Can you work these out from the model? Positions are in its coordinate system, mm. Face numbers are marked on the shaded views. Coordinates: 2 decimals unless noted, no trailing zeros. Write each loop counter-clockwise with the first axis right and the second up, starting at its lowest first coordinate (ties: lowest second). Pieces come first, ordered by that corner, then holes. Notation, with made-up numbers: (-2, 2) - (28, 2) arc R33 ccw to (28, 40) - close; hole circle Ø7 at (59, 23.5). An arc over 180 degrees is marked (long way). Use one line per item in the form item = value. Start each with the question number.
(1) If I drill on probe 1 along Y at (x, z) = (-29, 8); probe 2 along X at (y, z) = (11.5, 7.5); probe 3 along Z at (x, y) = (13, -8.5), over which ranges is the centre line in solid material (lowest first)? Write a range as from..to.
(2) If we section it at C-C on z = 12: Please give me the cut outline in (x, y), then the cut area to 3 significant figures.
(3) If we section it at A-A on z = 7.25: Give the number of separate pieces and of enclosed holes in the cut face, then the cut area to 3 significant figures.
(4) For pin 1 Ø3 at (y, z) = (17, 3.5) entering from -X; pin 2 Ø2 at (x, y) = (27.5, -15.5) entering from +Z; pin 3 Ø2 at (x, y) = (28.5, 11) entering from +Z; pin 4 Ø6 at (y, z) = (14.5, 13.5) entering from -X, each with a flat end and sliding along its axis, tell me the tip position at first contact or that it passes through.
(5) Thinking about a two-plate mould opening in X: for the marked faces 1, 2 and 3, which applies, pulls with the +X half, pulls with the -X half, needs draft (parallel to the pull), parting line crosses it, or undercut?
```python
from build123d import *

# Parameters (mm, degrees)
F2_DEPTH = 3
F1_R     = 2.5
F1_R_2   = 1.25
F3_DEPTH = 10
F4_SIZE2 = 3
F4_SIZE  = 2
F5_R     = 2.99999
F7_W     = 10
F7_H     = 18
F8_DEPTH = 4
F10_SIZE = 1


# Not quite as in the source:
# - a fillet or chamfer is up to 0.001 mm smaller than in the source, because OpenCascade refuses the exact size


with BuildPart() as f2:
    # F0 (on Top) → F2 (new body)
    with BuildSketch(Plane.XY):
        with BuildLine():
            ThreePointArc((46, 18), (43.0710678119, 25.0710678119), (36, 28))
            Line((36, 28), (-36, 28))
            ThreePointArc((-36, 28), (-43.0710678119, 25.0710678119), (-46, 18))
            Line((-46, 18), (-46, -18))
            ThreePointArc((-46, -18), (-43.0710678119, -25.0710678119), (-36, -28))
            Line((-36, -28), (36, -28))
            ThreePointArc((36, -28), (43.0710678119, -25.0710678119), (46, -18))
            Line((46, -18), (46, 18))
        make_face()
    extrude(amount=F2_DEPTH)

    # F1 (on Top) → F3 (join)
    with BuildSketch(Plane.XY):
        with Locations((-29, 11.5)):
            Circle(F1_R)
        with Locations((-29, 11.5)):
            Circle(F1_R_2, mode=Mode.SUBTRACT)
        with Locations((29, 11.5)):
            Circle(F1_R)
        with Locations((29, 11.5)):
            Circle(F1_R_2, mode=Mode.SUBTRACT)
        with Locations((-29, -11.5)):
            Circle(F1_R)
        with Locations((-29, -11.5)):
            Circle(F1_R_2, mode=Mode.SUBTRACT)
        with Locations((29, -11.5)):
            Circle(F1_R)
        with Locations((29, -11.5)):
            Circle(F1_R_2, mode=Mode.SUBTRACT)
    extrude(amount=F3_DEPTH)

    # F4
    f4_edges = [f2.edges().sort_by_distance(p)[0] for p in [
        (-31.5, 11.5, 3),
        (26.5, 11.5, 3),
        (26.5, -11.5, 3),
        (-31.5, -11.5, 3),
    ]]
    chamfer(f4_edges, length=F4_SIZE, length2=F4_SIZE2)

    # F5 (radius 3 in the source; OpenCascade refuses exactly that, so slightly less here)
    f5_edges = [f2.edges().sort_by_distance(p)[0] for p in [
        (0, 28, 3),
    ]]
    fillet(f5_edges, radius=F5_R)

    # F7 (on offset) → F8 (join)
    with BuildSketch(Plane.YZ.offset(46)):
        with Locations((0, 9)):
            Rectangle(F7_W, F7_H)
    extrude(amount=-F8_DEPTH)

    # F9: F2 across plane


with BuildPart() as f2_1:
    add(f2.part)
    add(f2.part.mirror(Plane.YZ))

    # F10
    f10_edges = [f2_1.edges().sort_by_distance(p)[0] for p in [
        (-46, 0, 18),
        (46, 0, 18),
    ]]
    chamfer(f10_edges, length=F10_SIZE)


solid = f2_1.part
```
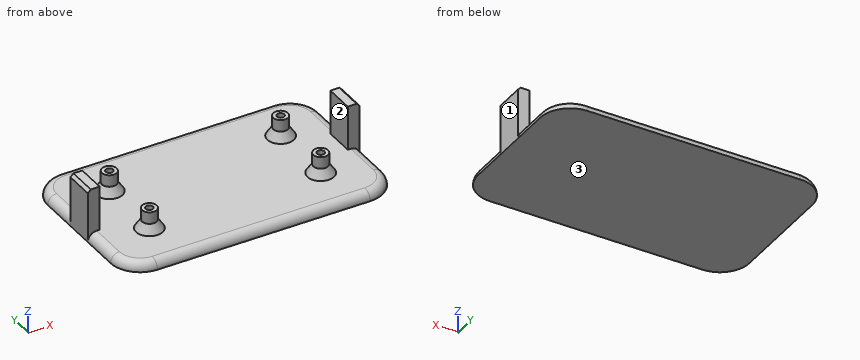
Reported:
q1.probe_1 = -14..-12.75, -10.25..-9, 9..10.25, 12.75..14
q1.probe_2 = -31.5..-30.25, -27.75..-26.5, 26.5..27.75, 30.25..31.5
q1.probe_3 = 0..3
q2.outline = (-46, -5) - (-42, -5) - (-42, 5) - (-46, 5) - close; (42, -5) - (46, -5) - (46, 5) - (42, 5) - close
q2.area = 80.0 mm2
q3.separate_pieces = 6
q3.enclosed_holes = 4
q3.area = 139 mm2
q4.pin_1 = -45.24
q4.pin_2 = 4.84
q4.pin_3 = 10
q4.pin_4 = through
q5.face_1 = pulls with the +X half
q5.face_2 = undercut
q5.face_3 = needs draft
